```python
from build123d import *

# Parameters (mm, degrees)
SKETCH1_R                      = 3.5
BOSS_EXTRUDE1_DEPTH            = 0.75
F_2_2_2_2_DIAMETER_HOLE1_D     = 2.2
F_3_2_3_2_DIAMETER_HOLE1_D     = 3.2
F_3_2_3_2_DIAMETER_HOLE1_DEPTH = 10
F_3_2_3_2_DIAMETER_HOLE1_TIP   = 0.96137699
CUT_EXTRUDE1_DEPTH             = 138.395414771
FILLET1_R                      = 2
SKETCH7_R                      = 4
CUT_EXTRUDE2_DEPTH             = 138.395414889


with BuildPart() as part:
    # Sketch1 → Boss-Extrude1 (new, symmetric)
    with BuildSketch(Plane(origin=(0, 0, 0), x_dir=(1, 0, 0), z_dir=(0, 1, 0))):
        with BuildLine():
            ThreePointArc((-41.13620668, -23.75), (-47.5, 0), (-41.13620668, 23.75))
            ThreePointArc((-41.13620668, 23.75), (-40.506696415, 24.5460597), (-39.675258631, 25.128043744))
            ThreePointArc((-39.675258631, 25.128043744), (-77.494729166, 13.448582828), (-117.056517742, 14.708361982))
            ThreePointArc((-117.056517742, 14.708361982), (-135, 0), (-117.056517742, -14.708361982))
            ThreePointArc((-117.056517742, -14.708361982), (-77.494729166, -13.448582828), (-39.675258631, -25.128043744))
            ThreePointArc((-39.675258631, -25.128043744), (-40.506696415, -24.5460597), (-41.13620668, -23.75))
        make_face()
        with BuildLine():
            ThreePointArc((-35.074028853, 20.25), (-39.855117767, 18.968911087), (-41.13620668, 23.75))
            ThreePointArc((-41.13620668, 23.75), (-47.5, 0), (-41.13620668, -23.75))
            ThreePointArc((-41.13620668, -23.75), (-39.855117767, -18.968911087), (-35.074028853, -20.25))
            ThreePointArc((-35.074028853, -20.25), (-40.5, 0), (-35.074028853, 20.25))
        make_face()
        with Locations((-38.105117767, -22)):
            Circle(SKETCH1_R)
        with Locations((-38.105117767, 22)):
            Circle(SKETCH1_R)
    extrude(amount=BOSS_EXTRUDE1_DEPTH, both=True)

    # Ø2.2 (2.2) Diameter Hole1 (through all)
    with Locations(Plane(origin=(0, 0.75, 0), x_dir=(1, 0, 0), z_dir=(0, 1, 0))):
        with Locations((-125.378942435, 5.51463095), (-114.418787327, 5.51463095), (-114.418787327, -5.445524158), (-125.378942435, -5.445524158)):
            Hole(F_2_2_2_2_DIAMETER_HOLE1_D / 2)

    # Ø3.2 (3.2) Diameter Hole1
    with Locations(Plane(origin=(0, 0.75, 0), x_dir=(1, 0, 0), z_dir=(0, 1, 0))):
        with Locations((-38.105117767, 22), (-38.105117767, -22), (-104.021186711, 9.323493222), (-104.021186711, -9.323493222)):
            Hole(F_3_2_3_2_DIAMETER_HOLE1_D / 2, depth=F_3_2_3_2_DIAMETER_HOLE1_DEPTH)
            with Locations((0, 0, -(F_3_2_3_2_DIAMETER_HOLE1_DEPTH + F_3_2_3_2_DIAMETER_HOLE1_TIP / 2))):  # 118° drill point
                Cone(0, F_3_2_3_2_DIAMETER_HOLE1_D / 2, F_3_2_3_2_DIAMETER_HOLE1_TIP, mode=Mode.SUBTRACT)

    # Sketch6 → Cut-Extrude1 (cut, through all)
    with BuildSketch(Plane(origin=(0, 0.75, 0), x_dir=(1, 0, 0), z_dir=(0, 1, 0))):
        with BuildLine():
            Line((-80.72687621, -6.02009961), (-55.965778938, 0))
            Line((-55.965778938, 0), (-80.72687621, 6.02009961))
            ThreePointArc((-80.72687621, 6.02009961), (-93.493210894, 5.375258779), (-106.259702082, 6.016993695))
            ThreePointArc((-106.259702082, 6.016993695), (-105, 0), (-106.259702082, -6.016993695))
            ThreePointArc((-106.259702082, -6.016993695), (-93.493210894, -5.375258779), (-80.72687621, -6.02009961))
        make_face()
        with BuildLine():
            Line((-70.096059807, 7.551982097), (-47.45584926, 2.047528026))
            ThreePointArc((-47.45584926, 2.047528026), (-46.716397825, 8.592332297), (-45.078723321, 14.971930527))
            ThreePointArc((-45.078723321, 14.971930527), (-57.396315368, 10.61771767), (-70.096059807, 7.551982097))
        make_face()
        with BuildLine():
            ThreePointArc((-45.078723321, -14.971930527), (-46.716397825, -8.592332297), (-47.45584926, -2.047528026))
            Line((-47.45584926, -2.047528026), (-70.096059807, -7.551982097))
            ThreePointArc((-70.096059807, -7.551982097), (-57.396315368, -10.61771767), (-45.078723321, -14.971930527))
        make_face()
    extrude(amount=-CUT_EXTRUDE1_DEPTH, mode=Mode.SUBTRACT)

    # Fillet1
    fillet1_edges = [part.edges().sort_by_distance(p)[0] for p in [
        (-47.45584926, 0, 2.047528026),
        (-45.078723321, 0, 14.971930527),
        (-70.096059807, 0, 7.551982097),
        (-106.259702082, 0, 6.016993695),
        (-106.259702082, 0, -6.016993695),
        (-80.72687621, 0, -6.02009961),
        (-55.965778938, 0, 0),
        (-80.72687621, 0, 6.02009961),
        (-45.078723321, 0, -14.971930527),
        (-47.45584926, 0, -2.047528026),
        (-70.096059807, 0, -7.551982097),
    ]]
    fillet(fillet1_edges, radius=FILLET1_R)

    # Sketch7 → Cut-Extrude2 (cut, through all)
    with BuildSketch(Plane(origin=(0, 0.75, 0), x_dir=(1, 0, 0), z_dir=(0, 1, 0))):
        with Locations(Location((-120, 0, 0), (0, 0, 270))):
            Circle(SKETCH7_R)
    extrude(amount=-CUT_EXTRUDE2_DEPTH, mode=Mode.SUBTRACT)


solid = part.part
```
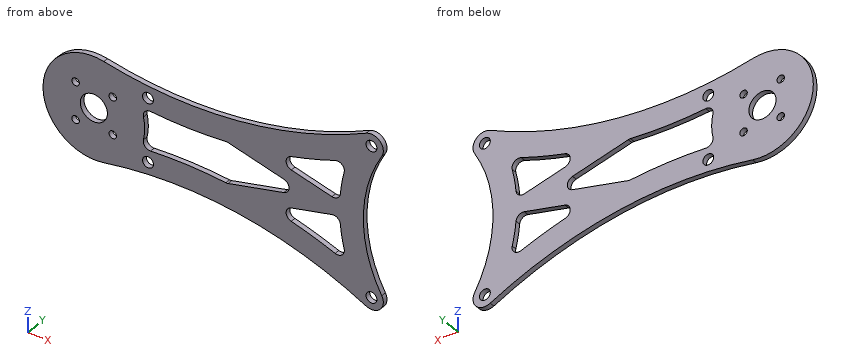
Part model, mm, in its own coordinate system. Round coordinates to 2 decimals unless told otherwise and drop trailing zeros. Order: outer loops, then holes, each group sorted by start corner. A loop starts at its lowest first (then second) coordinate and runs counter-clockwise, first axis right, second up. Notation, with made-up numbers: M 70,58.5 L 106,58.5 A8 ccw 106,67.5 Z; hole C 25,-14.5 d8. An arc over 180 degrees is marked long. Put each result on its own line as item: value. Start each with the question number.
1. Drill centre lines: probe 1 along Z at (x, y) = (-92.5, 0.6); probe 2 along Z at (x, y) = (-124.5, 0.3); probe 3 along X at (y, z) = (-0.55, 8). Where is each one in solid material? Low to high. Write a range as [from, to].
2. Slice it at B-B on z = 0. List the corners of the cut face in (x, y), then the cut area to 3 significant figures.
3. Slice it at A-A on x = -120. List the corners of the cut face in (y, z).
4. Drop a flat-ended pin along its axis: pin 1 (1.9 mm diameter, centred on x = -104.02, z = -9.32, fed in from +Y). Give the stop position or say it passes through.
5. Slice it at C-C on z = 22. List the corners of the cut face in (x, y), then the cut area to 3 significant figures.
6. Slice it at D-D on x = -57.5. List the corners of the cut face in (y, z), then the cut area to 3 significant figures.
Findings:
1. probe 1: [-12.38, -5.38], [5.38, 12.38]
1. probe 2: [-14.31, -6.18], [-4.85, 4.78], [6.11, 14.31]
1. probe 3: [-132.69, -104.92], [-103.12, -63.21], [-46.82, -39.7]
2. outline: M -135,-0.75 L -124,-0.75 L -124,0.75 L -135,0.75 Z; M -116,-0.75 L -105,-0.75 L -105,0.75 L -116,0.75 Z; M -62.43,-0.75 L -40.5,-0.75 L -40.5,0.75 L -62.43,0.75 Z
2. area: 65.9 mm2
3. outline: M -0.75,-15 L 0.75,-15 L 0.75,-4 L -0.75,-4 Z; M -0.75,4 L 0.75,4 L 0.75,15 L -0.75,15 Z
4. pin 1: through
5. outline: M -46.42,-0.75 L -39.71,-0.75 L -39.71,0.75 L -46.42,0.75 Z; M -36.51,-0.75 L -34.61,-0.75 L -34.61,0.75 L -36.51,0.75 Z
5. area: 12.9 mm2
6. outline: M -0.75,-17.91 L 0.75,-17.91 L 0.75,-10.59 L -0.75,-10.59 Z; M -0.75,-4.49 L 0.75,-4.49 L 0.75,4.49 L -0.75,4.49 Z; M -0.75,10.59 L 0.75,10.59 L 0.75,17.91 L -0.75,17.91 Z
6. area: 35.4 mm2
